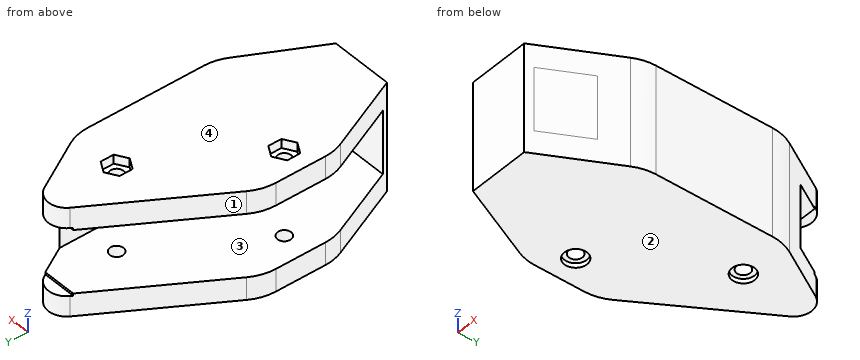
from build123d import *

# Parameters (mm, degrees)
SKETCH_1_W           = 41.838517058
SKETCH_1_H           = 61.659283987
SKETCH_1_R           = 1.5
EXTRUDE_1_DEPTH      = 24
SHELL_START          = 5
SHELL_2_OUTLINE_R    = 6.5
SHELL_2_DEPTH        = 14
SKETCH_7_W           = 14
SKETCH_7_H           = 61.659283987
CUT_EXTRUDE_2_DEPTH  = 38
SKETCH_11_W          = 14
SKETCH_11_H          = 61.659283987
EXTRUDE_2_DEPTH      = 14
SKETCH_12_W          = 10.1213772
SKETCH_12_H          = 61.659283987
CUT_EXTRUDE_3_DEPTH  = 52.896145639
CUT_EXTRUDE_5_DEPTH  = 47.819908548
SKETCH_18_W          = 15
SKETCH_18_H          = 18
CUT_EXTRUDE_6_DEPTH  = 54.011520411
EXTRUDE_5_DEPTH      = 24
SKETCH_22_W          = 27.838517058
SKETCH_22_H          = 14
CUT_EXTRUDE_8_DEPTH  = 17
SKETCH_23_W          = 14.991158549
SKETCH_23_H          = 11.73336261
EXTRUDE_8_DEPTH      = 2
FILLET_3_R           = 4
CUT_EXTRUDE_9_DEPTH  = 62.891048756
FILLET_4_R           = 4
FILLET_5_R           = 10
CUT_EXTRUDE_10_DEPTH = 2
SKETCH_26_R          = 2.5
CUT_EXTRUDE_11_DEPTH = 1


# Read off the part's stored shape, not the designer's step: 抽壳2
with BuildPart() as part:
    # 草图1 → 凸台-拉伸1 (new body)
    with BuildSketch(Plane.XY):
        with Locations((-8.896267572, -4.216675009)):
            Rectangle(SKETCH_1_W, SKETCH_1_H)
        with Locations((-8.896267572, -4.21667501)):
            Circle(SKETCH_1_R, mode=Mode.SUBTRACT)
        with Locations((6.176232993, -28.71667501)):
            Circle(SKETCH_1_R, mode=Mode.SUBTRACT)
    extrude(amount=EXTRUDE_1_DEPTH)

    # 抽壳2 outline → 抽壳2 (cut)
    # profile 1 of 2: a face of its own
    with BuildSketch(Plane.XY.offset(SHELL_START)):
        with BuildLine():
            Line((-24.815526101, 26.612966984), (-24.815526101, -35.046317003))
            Line((-24.815526101, -35.046317003), (4.697844602, -35.046317003))
            ThreePointArc((4.697844602, -35.046317003), (1.097738874, -24.659718332), (12.022990957, -25.876706469))
            Line((12.022990957, -25.876706469), (12.022990957, 26.612966984))
            Line((12.022990957, 26.612966984), (-24.815526101, 26.612966984))
        make_face()
        with Locations((-8.896267572, -4.21667501)):
            Circle(SHELL_2_OUTLINE_R, mode=Mode.SUBTRACT)
    # profile 2 of 2: a face of its own
    with BuildSketch(Plane.XY.offset(SHELL_START)):
        with BuildLine():
            ThreePointArc((12.022990957, -31.556643551), (10.23318967, -33.795169129), (7.654621384, -35.046317003))
            Line((7.654621384, -35.046317003), (12.022990957, -35.046317003))
            Line((12.022990957, -35.046317003), (12.022990957, -31.556643551))
        make_face()
    extrude(amount=SHELL_2_DEPTH, mode=Mode.SUBTRACT)

    # 草图7 → 切除-拉伸2 (cut)
    with BuildSketch(Plane(origin=(12.022990957, 0, 0), x_dir=(0, 0, -1), z_dir=(1, 0, 0))):
        with Locations((-12, -4.216675009)):
            Rectangle(SKETCH_7_W, SKETCH_7_H)
    extrude(amount=-CUT_EXTRUDE_2_DEPTH, mode=Mode.SUBTRACT)

    # 草图11 → 凸台-拉伸2 (add)
    with BuildSketch(Plane.ZY.offset(29.815526101)):
        with Locations((12, -4.216675009)):
            Rectangle(SKETCH_11_W, SKETCH_11_H)
    extrude(amount=-EXTRUDE_2_DEPTH)

    # 草图12 → 切除-拉伸3 (cut, through all)
    with BuildSketch(Plane.XY.offset(24)):
        with Locations((-24.754837501, -4.216675009)):
            Rectangle(SKETCH_12_W, SKETCH_12_H)
    extrude(amount=-CUT_EXTRUDE_3_DEPTH, mode=Mode.SUBTRACT)

    # 草图17 → 切除-拉伸5 (cut, through all)
    with BuildSketch(Plane.XY.offset(24)):
        Polygon((-8.896267572, 26.612966984), (-8.896267572, 14.867807771), (12.022990957, -19.135961659), (12.022990957, 26.612966984), align=None)
    extrude(amount=-CUT_EXTRUDE_5_DEPTH, mode=Mode.SUBTRACT)

    # 草图18 → 切除-拉伸6 (cut, through all)
    with BuildSketch(Plane.ZY.offset(19.694148901)):
        with Locations((12, 17.612966984)):
            Rectangle(SKETCH_18_W, SKETCH_18_H)
    extrude(amount=-CUT_EXTRUDE_6_DEPTH, mode=Mode.SUBTRACT)

    # 草图20 → 凸台-拉伸5 (add)
    with BuildSketch(Plane.XY.offset(24)):
        Polygon((-19.694148901, -35.046317003), (-9.853501275, -53.541034872), (3.683563025, -53.541034872), (12.022990957, -35.046317003), align=None)
    extrude(amount=-EXTRUDE_5_DEPTH)

    # 草图22 → 切除-拉伸8 (cut)
    with BuildSketch(Plane(origin=(0, -35.046317003, 0), x_dir=(1, 0, 0), z_dir=(0, 1, 0))):
        with Locations((-1.896267572, -12)):
            Rectangle(SKETCH_22_W, SKETCH_22_H)
    extrude(amount=-CUT_EXTRUDE_8_DEPTH, mode=Mode.SUBTRACT)

    # 草图23 → 凸台-拉伸8 (add)
    with BuildSketch(Plane(origin=(-29.881783728, -15.899464172, 0), x_dir=(0, 0, -1), z_dir=(0.8828123820911005, 0.469725768961675, 0))):
        with Locations((-11.904751729, -35.446570554)):
            Rectangle(SKETCH_23_W, SKETCH_23_H)
    extrude(amount=EXTRUDE_8_DEPTH)

    # 圆角3
    # the kernel refuses this fillet: 4 mm, written as the material it takes off along each edge
    with BuildSketch(Plane(origin=(-14.221722741, -41.073505124, 19), x_dir=(-0.8828123820904301, -0.4697257689629349, 0), z_dir=(0, 0, -1))) as fillet_3_piece_1:
        with BuildLine():
            CenterArc((4, -3.344189139), FILLET_3_R, 123.274953356, 56.725046644)
            Line((0, -3.344189139), (-0.08, -3.344189139))
            Line((-0.08, -3.344189139), (-0.08, 0))
            Line((-0.08, 0), (0, 0.08))
            ThreePointArc((0, 0.08), (0.902685209, 0.08), (1.761477827, 0.066883783))
            Line((1.761477827, 0.066883783), (1.805370419, 0))
        make_face()
    extrude(amount=14, mode=Mode.SUBTRACT)

    # 草图24 → 切除-拉伸9 (cut, through all)
    with BuildSketch(Plane(origin=(0, 0, 0), x_dir=(-1, 0, 0), z_dir=(0, 0, -1))):
        Polygon((8.896267572, 14.867807771), (19.694148901, -4.21667501), (19.694148901, 26.612966984), (8.896267572, 26.612966984), align=None)
    extrude(amount=-CUT_EXTRUDE_9_DEPTH, mode=Mode.SUBTRACT)

    # 圆角4
    fillet_4_edges = [part.edges().sort_by_distance(p)[0] for p in [
        (-8.896267572, 14.867807771, 2.25),
        (-8.896267572, 14.867807771, 21.75),
    ]]
    fillet(fillet_4_edges, radius=FILLET_4_R)

    # 圆角5
    fillet_5_edges = [part.edges().sort_by_distance(p)[0] for p in [
        (-19.694148901, -35.046317003, 12),
        (12.022990957, -19.135961659, 2.5),
        (12.022990957, -19.135961659, 21.5),
        (12.022990957, -35.046317003, 2.5),
        (-19.694148901, -4.21667501, 12),
        (12.022990957, -35.046317003, 21.5),
    ]]
    fillet(fillet_5_edges, radius=FILLET_5_R)

    # 草图25 → 切除-拉伸10 (cut)
    with BuildSketch(Plane.XY.offset(24)):
        Polygon((-8.896267572, -7.103426356), (-6.396267572, -5.660050683), (-6.396267572, -2.773299337), (-8.896267572, -1.329923664), (-11.396267572, -2.773299337), (-11.396267572, -5.660050683), align=None)
        Polygon((6.176232993, -25.829923664), (3.676232993, -27.273299337), (3.676232993, -30.160050683), (6.176232993, -31.603426356), (8.676232993, -30.160050683), (8.676232993, -27.273299337), align=None)
    extrude(amount=-CUT_EXTRUDE_10_DEPTH, mode=Mode.SUBTRACT)

    # 草图26 → 切除-拉伸11 (cut)
    with BuildSketch(Plane(origin=(0, 0, 0), x_dir=(-1, 0, 0), z_dir=(0, 0, -1))):
        with Locations((8.896267572, -4.21667501)):
            Circle(SKETCH_26_R)
        with Locations((-6.176232993, -28.71667501)):
            Circle(SKETCH_26_R)
    extrude(amount=-CUT_EXTRUDE_11_DEPTH, mode=Mode.SUBTRACT)


with BuildPart() as body_2:
    # 镜向1: mirrored copy
    add(part.part.mirror(Plane.ZY.offset(29.694148901)))


solid = body_2.part
Geometry check sheet. Reference: the model listing, model coordinates, mm. Face numbers are marked on the shaded views. Give positions to 0.01 mm unless a question says otherwise; leave off trailing zeros. Order: outer loops, then holes, each group sorted by start corner. A loop starts at its lowest first (then second) coordinate and runs counter-clockwise, first axis right, second up.
1) Cross-section at A-A (y = -14.5). Record the boundary of the cut face in (x, z), then the cut area to 3 significant figures.
Results are:
outline: (-68.56, 0) - (-39.69, 0) - (-39.69, 24) - (-68.56, 24) - (-68.56, 19) - (-43.57, 19) - (-43.57, 5) - (-68.56, 5) - close
area: 343 mm2
2) Cross-section at D-D (x = -42.5). Record the boundary of the cut face in (y, z).
Results are:
outline: (-40.32, 0) - (0.74, 0) - (0.74, 24) - (-40.32, 24) - close
3) Cross-section at C-C (x = -59.5). Record the boundary of the cut face in (y, z), then the cut area to 3 significant figures.
Results are:
outline: (-53.54, 0) - (0.23, 0) - (0.23, 5) - (-52.05, 5) - (-52.05, 19) - (0.23, 19) - (0.23, 24) - (-53.54, 24) - close
area: 559 mm2
4) Material ranges on probe 1 along Z at (x, y) = (-65, -47); probe 2 along Y at (x, z) = (-53.5, 13.75); probe 3 along X at (y, z) = (-7, 10.5), recorded low to high.
Results are:
probe 1: z = 0 to 5, 19 to 24
probe 2: y = -53.54 to -52.05
probe 3: x = -43.57 to -39.69
5) Gauge pin test, flat ends, axial feed: pin 1 (5 mm diameter, centred on x = -57.5, z = 11.5, fed in from +Y); pin 2 (0.6 mm diameter, centred on y = -5, z = 22.5, fed in from +X); pin 3 (4 mm diameter, centred on x = -65.56, y = -28.72, fed in from -Z). Record the tip position at first contact, or that the pin passes through.
Results are:
pin 1: stops at y = -52.05
pin 2: stops at x = -39.81
pin 3: stops at z = 1
6) Cross-section at B-B (z = 10.25). Record the boundary of the cut face in (x, y), then the cut area to 3 significant figures.
Results are:
outline: (-63.75, -52.05) - (-63.07, -53.54) - (-49.53, -53.54) - (-40.87, -37.25) arc R10 ccw to (-39.69, -32.55) - (-39.69, -6.85) arc R10 ccw to (-40.99, -1.93) - (-43.57, 2.64) - (-43.57, -41.92) arc R4 ccw to (-46.74, -44.03) - (-50.68, -51.43) - (-49.52, -52.05) - close
area: 189 mm2
7) Draft check along Z on the marked faces 1, 2, 3 and 4. Enter one of: released by +Z, released by -Z, zero draft, split by the parting line, or undercut.
Results are:
face 1: zero draft
face 2: released by -Z
face 3: undercut
face 4: released by +Z
